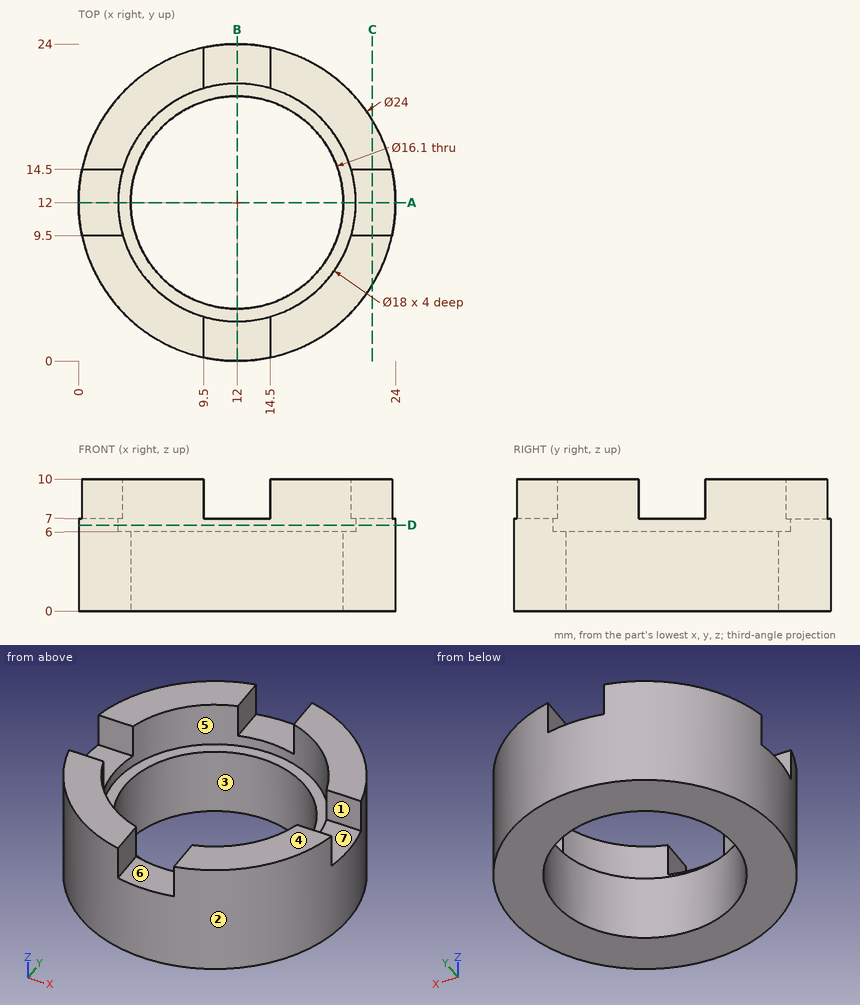
The drawing under review shows one solid part. Ordinate dimensions are in mm from its lowest x, y, z. A direction names the side the tool comes from. Round coordinates to 2 decimals unless told otherwise and drop trailing zeros. Loops run counter-clockwise (first coordinate to the right, second up) from the corner with the lowest first, then second, coordinate; pieces in that order, holes last. Notation, with made-up numbers: M 84.25,72 L 134.25,72 A29 ccw 134.25,108 Z; hole C 69,-38 d3. An arc over 180 degrees is marked long. Answer as CSV lines item,"result". Start each with the question number.
Item 1: Wall thickness on line 1 (Y direction, x = 12, z = 3.2); line 2 (Z direction, x = 22.75, y = 11.75); line 3 (X direction, y = 4.75, z = 8.5): over which ranges is each line inside the solid? List them lowest first. Write a range as [from, to].
Item 2: Consider section C-C (x = 22.25). Write out the cut boundary in (y, z).
Item 3: Consider section D-D (z = 6.5). Write out the cut boundary in (x, y), then the cut area to 3 significant figures.
Item 4: Insertion check: P1, Ø6, axis at x = 19, z = 7, coming from the -Y side; P2, Ø0.9, axis at y = 2.5, z = 8.5, coming from the -X side; P3, Ø1.5, axis at x = 1.5, z = 8.5, coming from the +Y side. Each pin has a flat end and moves straight along its axis. Give the tip position at first contact, or say it passes through.
Item 5: Mouldability with a two-part tool opening along Y and no side actions: class the marked faces 1, 2, 3 and 4 as released by +Y, released by -Y, zero draft, split by the parting line, or undercut.
Item 6: Consider section A-A (y = 12). Write out the cut boundary in (x, z), then the cut area to 3 significant figures.
Item 7: For the marked faces 5, 6 and 7, list the 3-axis set-ups (+Z, -Z, +X, -X, +Y, -Y) from which the entire face can be reached by the end or side of a thin tool; tool diameter is ignored.
Answer:
1,line 1,"y = [0, 3.95], [20.05, 24]"
1,line 2,"z = [0, 7]"
1,line 3,"x = [2.44, 6.67], [17.33, 21.56]"
2,outline,"M 5.76,0 L 18.24,0 L 18.24,10 L 14.5,10 L 14.5,7 L 9.5,7 L 9.5,10 L 5.76,10 Z"
3,outline,"C 12,12 d24; hole C 12,12 d18"
3,area,"198 mm^2"
4,P1,"stops at y = 0.69"
4,P2,"stops at x = 4.12"
4,P3,"stops at y = 19"
5,face 1,"undercut"
5,face 2,"split by the parting line"
5,face 3,"undercut"
5,face 4,"zero draft"
6,outline,"M 0,0 L 3.95,0 L 3.95,6 L 3,6 L 3,7 L 0,7 Z; M 20.05,0 L 24,0 L 24,7 L 21,7 L 21,6 L 20.05,6 Z"
6,area,"53.4 mm^2"
7,face 5,"+Z"
7,face 6,"+Z, +Y, -Y"
7,face 7,"+Z, +X, -X"
